```python
from build123d import *

# Parameters (mm, degrees)
BOSS_EXTRUDE1_DEPTH     = 38
CUT_EXTRUDE1_DEPTH      = 78.345006303
CUT_EXTRUDE1_DEPTH_BACK = 78.345006303
SKETCH2_OUTSIDE_W       = 105.518
SKETCH2_OUTSIDE_H       = 143.018
SHELL1_START            = -13.5
SHELL1_DEPTH            = 13.5
CUT_EXTRUDE2_DEPTH      = 78.345006303
CUT_EXTRUDE2_DEPTH_BACK = 78.345006303
SKETCH3_R               = 2.5
CUT_EXTRUDE3_DEPTH      = 38
SKETCH5_R               = 2.5
BOSS_EXTRUDE2_DEPTH     = 0.5
LPATTERN1_COUNT         = 3
LPATTERN1_PITCH         = 17.5
SKETCH7_W               = 70
SKETCH7_H               = 64.783051232
BOSS_EXTRUDE3_DEPTH     = 3


# Read off the part's stored shape, not the designer's step: Shell1
with BuildPart() as part:
    # Sketch1 → Boss-Extrude1 (new, symmetric)
    with BuildSketch(Plane(origin=(0, 0, 0), x_dir=(0, 0, -1), z_dir=(1, 0, 0))):
        with BuildLine():
            Line((-61, 0), (-66, 0))
            Line((-66, 0), (-66, 3))
            Line((-66, 3), (47.5, 3))
            Line((47.5, 3), (47.5, 0))
            Line((47.5, 0), (36.207291717, -13.5))
            Line((36.207291717, -13.5), (-47.5, -13.5))
            ThreePointArc((-47.5, -13.5), (-57.045941546, -9.545941546), (-61, 0))
        make_face()
    extrude(amount=BOSS_EXTRUDE1_DEPTH, both=True)

    # Sketch2 outside → Cut-Extrude1 (cut, two sides: drawn at the far end of the back side and taken through both)
    with BuildSketch(Plane(origin=(0, 0, 0), x_dir=(1, 0, 0), z_dir=(0, 1, 0)).offset(-CUT_EXTRUDE1_DEPTH_BACK)):
        with Locations((0, -9.25)):
            Rectangle(SKETCH2_OUTSIDE_W, SKETCH2_OUTSIDE_H)
        Polygon((-25, -66), (-38, -61), (-38, 36.207291717), (-20, 47.5), (20, 47.5), (38, 36.207291717), (38, -61), (25, -66), align=None, mode=Mode.SUBTRACT)
    extrude(amount=CUT_EXTRUDE1_DEPTH + CUT_EXTRUDE1_DEPTH_BACK, mode=Mode.SUBTRACT)

    # Shell1 outline → Shell1 (cut)
    with BuildSketch(Plane(origin=(0, 0, 0), x_dir=(1, 0, 0), z_dir=(0, 1, 0)).offset(SHELL1_START)):
        Polygon((19.136843791, 44.5), (-19.136843791, 44.5), (-35, 34.547889139), (-35, -68), (35, -68), (35, 34.547889139), align=None)
    extrude(amount=SHELL1_DEPTH, mode=Mode.SUBTRACT)

    # Sketch3 → Cut-Extrude2 (cut, two sides: drawn at the far end of the back side and taken through both)
    with BuildSketch(Plane(origin=(0, 0, 0), x_dir=(0, 0, -1), z_dir=(1, 0, 0)).offset(-CUT_EXTRUDE2_DEPTH_BACK)):
        with Locations((-47.5, -6.75)):
            Circle(SKETCH3_R)
    extrude(amount=CUT_EXTRUDE2_DEPTH + CUT_EXTRUDE2_DEPTH_BACK, mode=Mode.SUBTRACT)

    # Sketch4 → Cut-Extrude3 (cut)
    with BuildSketch(Plane(origin=(0, 0, 0), x_dir=(0, 0, -1), z_dir=(1, 0, 0))):
        Polygon((-22.5, 0), (47.5, 0), (36.207291717, -13.5), (-33.792708283, -13.5), align=None)
    extrude(amount=CUT_EXTRUDE3_DEPTH, mode=Mode.SUBTRACT)

    # Sketch5 → Boss-Extrude2 (add, symmetric)
    with BuildSketch(Plane(origin=(17.5, 0, 0), x_dir=(0, 0, -1), z_dir=(1, 0, 0))):
        with BuildLine():
            Line((-61, 0), (-32.281378795, 0))
            Line((-32.281378795, 0), (-43.618023888, -13.5))
            Line((-43.618023888, -13.5), (-47.5, -13.5))
            ThreePointArc((-47.5, -13.5), (-57.045941546, -9.545941546), (-61, 0))
        make_face()
        with Locations((-47.5, -6.75)):
            Circle(SKETCH5_R, mode=Mode.SUBTRACT)
    boss_extrude2 = extrude(amount=BOSS_EXTRUDE2_DEPTH, both=True)

    # LPattern1: Boss-Extrude2 ×3
    with Locations(*[(-i * LPATTERN1_PITCH, 0, 0) for i in range(1, LPATTERN1_COUNT)]):
        add(boss_extrude2)

    # Sketch7 → Boss-Extrude3 (add)
    with BuildSketch(Plane.XZ):
        with Locations((0, -1.970822706)):
            Rectangle(SKETCH7_W, SKETCH7_H)
    extrude(amount=BOSS_EXTRUDE3_DEPTH)


solid = part.part
```
Can you work these out from the model? Positions are in its coordinate system, mm. A direction names the side the tool comes from. Give positions to 0.01 mm unless a question says otherwise; leave off trailing zeros. Write each loop counter-clockwise with the first axis right and the second up, starting at its lowest first coordinate (ties: lowest second). Pieces come first, ordered by that corner, then holes. Notation, with made-up numbers: (7.25, 77.5) -> (53.25, 77.5) arc R21 cw to (53.25, 82.5) -> close; hole circle Ø7 at (32.25, 81). An arc over 180 degrees is marked (long way). Write item = value, one per line.
(1) For faces 1 (the face through (38, -3, 33)), 2 (the face through (-9, -2, -44.5)), 3 (the face through (35, -1, -5)), 4 (the face through (36.52, -9.65, 56.94)), 5 (the face through (17, -5, 50)), which set-ups out of +Z, -Z, +X, -X, +Y, -Y let a thin tool reach every point of the face, with its end or its side?
Worked out:
face_1 = +Z, -Z, +X, +Y, -Y
face_2 = +X, -Y
face_3 = -Z, +X, -Y
face_4 = +Z, +X, -X, -Y
face_5 = +Z, -Y
(2) Suppose I cut it at C-C on x = 12. Write out the boundary of the cut face in (y, z), then the cut area to 3 significant figures.
Worked out:
outline = (-3, -34.36) -> (0, -34.36) -> (0, -47.5) -> (3, -47.5) -> (3, 66) -> (0, 66) -> (0, 30.42) -> (-3, 30.42) -> close
area = 535 mm^2
(3) I'm going to push flat-ended pins straight in: P1, Ø4, axis at x = 4, z = 17.5, coming from the -Y side; P2, Ø8, axis at x = -2, y = -1.5, coming from the +Z side; P3, Ø1.5, axis at y = -1, z = -5.5, coming from the +X side; P4, Ø1.5, axis at x = 14, y = -1, coming from the -Z side. Where does each tip first touch, or does it pass through?
Worked out:
P1 = -3
P2 = 66
P3 = 35
P4 = -34.36
(4) Suppose I cut it at A-A on x = -3. Write out the boundary of the cut face in (y, z).
Worked out:
outline = (-3.59, -44.5) -> (0, -47.5) -> (3, -47.5) -> (3, 66) -> (0, 66) -> (0, 30.42) -> (-3, 30.42) -> (-3, -34.36) -> (0, -34.36) -> (0, -44.5) -> close
(5) Suppose I cut it at B-B on z = 4. Write out the boundary of the cut face in (x, y), then the cut area to 4 significant figures.
Worked out:
outline = (-38, -13.5) -> (-35, -13.5) -> (-35, -3) -> (35, -3) -> (35, 0) -> (38, 0) -> (38, 3) -> (-38, 3) -> close
area = 478.5 mm^2
(6) Suppose I cut it at D-D on y = -6.75. Count the separate pieces of the cut face and the enclosed holes in it, then the cut area to 3 significant figures.
Worked out:
separate_pieces = 10
enclosed_holes = 0
area = 432 mm^2
(7) Thinking about a two-plate mould opening in Y: for faces 6 (the face through (-31.409, 1.479, 63.535)), 7 (the face through (17.51, -9.65, 56.94)), 8 (the face through (-17.51, -7.71, 45.19)), which applies, released by +Y, released by -Y, zero draft, split by the parting line, or undercut?
Worked out:
face_6 = zero draft
face_7 = released by -Y
face_8 = undercut
(8) I need wall thicknesses on probe 1 along X at (y, z) = (-1.5, 44); probe 2 along Y at (x, z) = (35.7, 47.5); probe 3 along X at (y, z) = (-7.25, -13). Which ranges of each line are inside material? Lowest first, please. Write a range as from..to.
Worked out:
probe_1 = -38..-35, -18..-17, -0.5..0.5, 17..18, 35..38
probe_2 = -13.5..-9.25, -4.25..3
probe_3 = -38..-35
